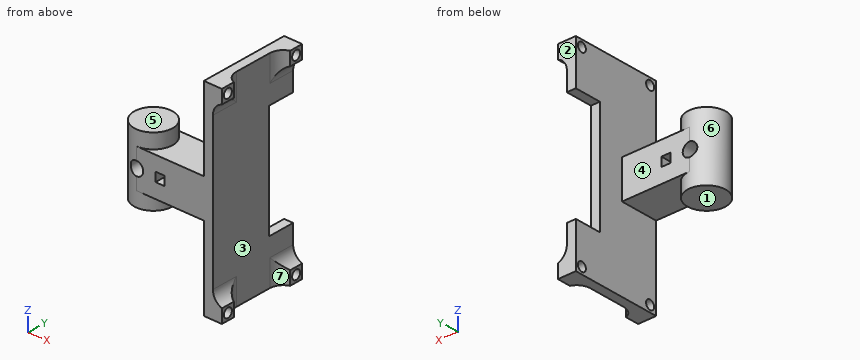
from build123d import *

# Parameters (mm, degrees)
SKETCH1_R               = 4.25
BOSS_EXTRUDE1_DEPTH     = 7.5
SKETCH2_W               = 8.5
SKETCH2_H               = 8.5
BOSS_EXTRUDE2_DEPTH     = 15
SKETCH3_W               = 45
SKETCH3_H               = 20
BOSS_EXTRUDE3_DEPTH     = 4
SKETCH4_R               = 1
CUT_EXTRUDE1_DEPTH      = 36.984371608
CUT_EXTRUDE2_DEPTH      = 2
SKETCH6_W               = 25
SKETCH6_H               = 6
CUT_EXTRUDE3_DEPTH      = 2
CUT_EXTRUDE4_DEPTH      = 32.614869919
CUT_EXTRUDE4_DEPTH_BACK = 32.614869919
SKETCH7_R               = 1.5
CUT_EXTRUDE5_DEPTH      = 34.396294705
CUT_EXTRUDE5_DEPTH_BACK = 34.396294705
SKETCH8_W               = 2
SKETCH8_H               = 2
FILLET1_R               = 3


with BuildPart() as part:
    # Sketch1 → Boss-Extrude1 (new, symmetric)
    with BuildSketch(Plane.XY):
        Circle(SKETCH1_R)
    extrude(amount=BOSS_EXTRUDE1_DEPTH, both=True)

    # Sketch2 → Boss-Extrude2 (add)
    with BuildSketch(Plane(origin=(0, 0, 0), x_dir=(0, 0, -1), z_dir=(1, 0, 0))):
        Rectangle(SKETCH2_W, SKETCH2_H)
    extrude(amount=BOSS_EXTRUDE2_DEPTH)

    # Sketch3 → Boss-Extrude3 (add)
    with BuildSketch(Plane(origin=(15, 0, 0), x_dir=(0, 0, -1), z_dir=(1, 0, 0))):
        with Locations((0, 5.75)):
            Rectangle(SKETCH3_W, SKETCH3_H)
    extrude(amount=BOSS_EXTRUDE3_DEPTH)

    # Sketch4 → Cut-Extrude1 (cut, through all)
    with BuildSketch(Plane(origin=(19, 0, 0), x_dir=(0, 0, -1), z_dir=(1, 0, 0))):
        with Locations((-21, 14.25)):
            Circle(SKETCH4_R)
        with Locations((-21, -2.75)):
            Circle(SKETCH4_R)
        with Locations((21, -2.75)):
            Circle(SKETCH4_R)
        with Locations((21, 14.25)):
            Circle(SKETCH4_R)
    extrude(amount=-CUT_EXTRUDE1_DEPTH, mode=Mode.SUBTRACT)

    # Sketch5 → Cut-Extrude2 (cut)
    with BuildSketch(Plane(origin=(19, 0, 0), x_dir=(0, 0, -1), z_dir=(1, 0, 0))):
        Polygon((19.5, 15.75), (-19.5, 15.75), (-19.5, 12.75), (-22.5, 12.75), (-22.5, -1.25), (-19.5, -1.25), (-19.5, -4.25), (19.5, -4.25), (19.5, -1.25), (22.5, -1.25), (22.5, 12.75), (19.5, 12.75), align=None)
    extrude(amount=-CUT_EXTRUDE2_DEPTH, mode=Mode.SUBTRACT)

    # Sketch6 → Cut-Extrude3 (cut)
    with BuildSketch(Plane(origin=(17, 0, 0), x_dir=(0, 0, -1), z_dir=(1, 0, 0))):
        with Locations((0, 12.75)):
            Rectangle(SKETCH6_W, SKETCH6_H)
    extrude(amount=-CUT_EXTRUDE3_DEPTH, mode=Mode.SUBTRACT)

    # Sketch7 → Cut-Extrude4 (cut, two sides: drawn at the far end of the back side and taken through both)
    with BuildSketch(Plane(origin=(0, 4.25, 0), x_dir=(1, 0, 0), z_dir=(0, 1, 0)).offset(-CUT_EXTRUDE4_DEPTH_BACK)):
        with Locations(Location((0, 0, 0), (0, 0, 270))):
            Circle(SKETCH7_R)
    extrude(amount=CUT_EXTRUDE4_DEPTH + CUT_EXTRUDE4_DEPTH_BACK, mode=Mode.SUBTRACT)

    # Sketch8 → Cut-Extrude5 (cut, two sides: drawn at the far end of the back side and taken through both)
    with BuildSketch(Plane(origin=(0, 0, 0), x_dir=(1, 0, 0), z_dir=(0, 1, 0)).offset(-CUT_EXTRUDE5_DEPTH_BACK)):
        with Locations((5.25, 0)):
            Rectangle(SKETCH8_W, SKETCH8_H)
    extrude(amount=CUT_EXTRUDE5_DEPTH + CUT_EXTRUDE5_DEPTH_BACK, mode=Mode.SUBTRACT)

    # Fillet1
    # the kernel refuses this fillet: 3 mm, written as the material it adds along each edge
    with BuildSketch(Plane(origin=(17, -1.25, -19.5), x_dir=(0, 1, 0), z_dir=(0, 0, -1)), Plane(origin=(17, -4.25, -19.5), x_dir=(0, 0, 1), z_dir=(0, 1, 0)), Plane(origin=(17, 12.75, -19.5), x_dir=(0, 0, 1), z_dir=(0, 1, 0)), Plane(origin=(17, 12.75, -22.5), x_dir=(0, -1, 0), z_dir=(0, 0, 1)), Plane(origin=(17, -1.25, 22.5), x_dir=(0, 1, 0), z_dir=(0, 0, -1)), Plane(origin=(17, 15.75, 19.5), x_dir=(0, 0, -1), z_dir=(0, -1, 0)), Plane(origin=(17, 12.75, 19.5), x_dir=(0, -1, 0), z_dir=(0, 0, 1))) as fillet1_piece_1:
        with BuildLine():
            CenterArc((2.828427125, 3), FILLET1_R, 199.471220634, 70.528779366)
            Line((0, 2), (-0.056568542, 1.98))
            ThreePointArc((-0.056568542, 1.98), (-0.06, 1), (-0.06, 0))
            Line((-0.06, 0), (0, -0.06))
            Line((0, -0.06), (2.828427125, -0.06))
            Line((2.828427125, -0.06), (2.828427125, 0))
        make_face()
    extrude(amount=3)
    with BuildSketch(Plane(origin=(17, -1.25, 19.5), x_dir=(1, 0, 0), z_dir=(0, -1, 0))) as fillet1_piece_2:
        with BuildLine():
            CenterArc((3, -2.828427125), FILLET1_R, 109.471220634, 70.528779366)
            Line((0, -2.828427125), (-0.06, -2.828427125))
            Line((-0.06, -2.828427125), (-0.06, 0))
            Line((-0.06, 0), (0, 0.06))
            ThreePointArc((0, 0.06), (1, 0.06), (1.98, 0.056568542))
            Line((1.98, 0.056568542), (2, 0))
        make_face()
    extrude(amount=3)
    with BuildSketch(Plane(origin=(17, -1.25, -12.428932188), x_dir=(0, 1, 0), z_dir=(0, 0, -1))) as fillet1_piece_3a_section:
        with BuildLine():
            CenterArc((2.828427125, 3), FILLET1_R, 199.471220634, 70.528779366)
            Line((0, 2), (-0.056568542, 1.98))
            ThreePointArc((-0.056568542, 1.98), (-0.06, 1), (-0.06, 0))
            Line((-0.06, 0), (0, -0.06))
            Line((0, -0.06), (2.828427125, -0.06))
            Line((2.828427125, -0.06), (2.828427125, 0))
        make_face()
    fillet1_piece_3a = extrude(amount=10.071067812, mode=Mode.PRIVATE)
    fillet1_piece_3a = split(fillet1_piece_3a, bisect_by=Plane(origin=(17.51353179, -0.571681569, -19.5), z_dir=(0, 0, 1)), keep=Keep.TOP, mode=Mode.PRIVATE)
    with BuildSketch(Plane(origin=(17, -4.25, -19.5), x_dir=(0, 0, 1), z_dir=(0, 1, 0))) as fillet1_piece_3b_section:
        with BuildLine():
            CenterArc((2.828427125, 3), FILLET1_R, 199.471220634, 70.528779366)
            Line((0, 2), (-0.056568542, 1.98))
            ThreePointArc((-0.056568542, 1.98), (-0.06, 1), (-0.06, 0))
            Line((-0.06, 0), (0, -0.06))
            Line((0, -0.06), (2.828427125, -0.06))
            Line((2.828427125, -0.06), (2.828427125, 0))
        make_face()
    fillet1_piece_3b = extrude(amount=10.071067812, mode=Mode.PRIVATE)
    fillet1_piece_3b = split(fillet1_piece_3b, bisect_by=Plane(origin=(17.51353179, -1.25, -18.821681569), z_dir=(0, 1, 0)), keep=Keep.TOP, mode=Mode.PRIVATE)
    fillet1_piece_3 = fillet1_piece_3a & fillet1_piece_3b
    add(fillet1_piece_3)
    with BuildSketch(Plane(origin=(17, 5.678932188, -19.5), x_dir=(0, 0, 1), z_dir=(0, 1, 0))) as fillet1_piece_4a_section:
        with BuildLine():
            CenterArc((2.828427125, 3), FILLET1_R, 199.471220634, 70.528779366)
            Line((0, 2), (-0.056568542, 1.98))
            ThreePointArc((-0.056568542, 1.98), (-0.06, 1), (-0.06, 0))
            Line((-0.06, 0), (0, -0.06))
            Line((0, -0.06), (2.828427125, -0.06))
            Line((2.828427125, -0.06), (2.828427125, 0))
        make_face()
    fillet1_piece_4a = extrude(amount=10.071067812, mode=Mode.PRIVATE)
    fillet1_piece_4a = split(fillet1_piece_4a, bisect_by=Plane(origin=(17.51353179, 12.75, -18.821681569), z_dir=(0, -1, 0)), keep=Keep.TOP, mode=Mode.PRIVATE)
    with BuildSketch(Plane(origin=(17, 12.75, -22.5), x_dir=(0, -1, 0), z_dir=(0, 0, 1))) as fillet1_piece_4b_section:
        with BuildLine():
            CenterArc((2.828427125, 3), FILLET1_R, 199.471220634, 70.528779366)
            Line((0, 2), (-0.056568542, 1.98))
            ThreePointArc((-0.056568542, 1.98), (-0.06, 1), (-0.06, 0))
            Line((-0.06, 0), (0, -0.06))
            Line((0, -0.06), (2.828427125, -0.06))
            Line((2.828427125, -0.06), (2.828427125, 0))
        make_face()
    fillet1_piece_4b = extrude(amount=10.071067812, mode=Mode.PRIVATE)
    fillet1_piece_4b = split(fillet1_piece_4b, bisect_by=Plane(origin=(17.51353179, 12.071681569, -12.5), z_dir=(0, 0, -1)), keep=Keep.TOP, mode=Mode.PRIVATE)
    fillet1_piece_4b = split(fillet1_piece_4b, bisect_by=Plane(origin=(17.51353179, 12.071681569, -19.5), z_dir=(0, 0, 1)), keep=Keep.TOP, mode=Mode.PRIVATE)
    fillet1_piece_4 = fillet1_piece_4a & fillet1_piece_4b
    add(fillet1_piece_4)
    with BuildSketch(Plane(origin=(17, 5.821067812, 19.5), x_dir=(1, 0, 0), z_dir=(0, -1, 0))) as fillet1_piece_5a_section:
        with BuildLine():
            CenterArc((3, -2.828427125), FILLET1_R, 109.471220634, 70.528779366)
            Line((0, -2.828427125), (-0.06, -2.828427125))
            Line((-0.06, -2.828427125), (-0.06, 0))
            Line((-0.06, 0), (0, 0.06))
            ThreePointArc((0, 0.06), (1, 0.06), (1.98, 0.056568542))
            Line((1.98, 0.056568542), (2, 0))
        make_face()
    fillet1_piece_5a = extrude(amount=10.071067812, mode=Mode.PRIVATE)
    fillet1_piece_5a = split(fillet1_piece_5a, bisect_by=Plane(origin=(17.51353179, -1.25, 18.821681569), z_dir=(0, 1, 0)), keep=Keep.TOP, mode=Mode.PRIVATE)
    with BuildSketch(Plane(origin=(17, -1.25, 22.5), x_dir=(0, 1, 0), z_dir=(0, 0, -1))) as fillet1_piece_5b_section:
        with BuildLine():
            CenterArc((2.828427125, 3), FILLET1_R, 199.471220634, 70.528779366)
            Line((0, 2), (-0.056568542, 1.98))
            ThreePointArc((-0.056568542, 1.98), (-0.06, 1), (-0.06, 0))
            Line((-0.06, 0), (0, -0.06))
            Line((0, -0.06), (2.828427125, -0.06))
            Line((2.828427125, -0.06), (2.828427125, 0))
        make_face()
    fillet1_piece_5b = extrude(amount=10.071067812, mode=Mode.PRIVATE)
    fillet1_piece_5b = split(fillet1_piece_5b, bisect_by=Plane(origin=(17.51353179, -0.571681569, 19.5), z_dir=(0, 0, -1)), keep=Keep.TOP, mode=Mode.PRIVATE)
    fillet1_piece_5 = fillet1_piece_5a & fillet1_piece_5b
    add(fillet1_piece_5)
    with BuildSketch(Plane(origin=(17, 12.75, 12.428932188), x_dir=(0, -1, 0), z_dir=(0, 0, 1))) as fillet1_piece_6a_section:
        with BuildLine():
            CenterArc((2.828427125, 3), FILLET1_R, 199.471220634, 70.528779366)
            Line((0, 2), (-0.056568542, 1.98))
            ThreePointArc((-0.056568542, 1.98), (-0.06, 1), (-0.06, 0))
            Line((-0.06, 0), (0, -0.06))
            Line((0, -0.06), (2.828427125, -0.06))
            Line((2.828427125, -0.06), (2.828427125, 0))
        make_face()
    fillet1_piece_6a = extrude(amount=10.071067812, mode=Mode.PRIVATE)
    fillet1_piece_6a = split(fillet1_piece_6a, bisect_by=Plane(origin=(17.51353179, 12.071681569, 12.5), z_dir=(0, 0, 1)), keep=Keep.TOP, mode=Mode.PRIVATE)
    fillet1_piece_6a = split(fillet1_piece_6a, bisect_by=Plane(origin=(17.51353179, 12.071681569, 19.5), z_dir=(0, 0, -1)), keep=Keep.TOP, mode=Mode.PRIVATE)
    with BuildSketch(Plane(origin=(17, 15.75, 19.5), x_dir=(0, 0, -1), z_dir=(0, -1, 0))) as fillet1_piece_6b_section:
        with BuildLine():
            CenterArc((2.828427125, 3), FILLET1_R, 199.471220634, 70.528779366)
            Line((0, 2), (-0.056568542, 1.98))
            ThreePointArc((-0.056568542, 1.98), (-0.06, 1), (-0.06, 0))
            Line((-0.06, 0), (0, -0.06))
            Line((0, -0.06), (2.828427125, -0.06))
            Line((2.828427125, -0.06), (2.828427125, 0))
        make_face()
    fillet1_piece_6b = extrude(amount=10.071067812, mode=Mode.PRIVATE)
    fillet1_piece_6b = split(fillet1_piece_6b, bisect_by=Plane(origin=(17.51353179, 12.75, 18.821681569), z_dir=(0, -1, 0)), keep=Keep.TOP, mode=Mode.PRIVATE)
    fillet1_piece_6 = fillet1_piece_6a & fillet1_piece_6b
    add(fillet1_piece_6)


solid = part.part
The listing builds one solid part. Answer for the finished solid, in the listing's coordinates (mm). Face numbers are marked on the shaded views. A direction names the side the tool comes from. Give positions to 0.01 mm unless a question says otherwise; leave off trailing zeros. Write each loop counter-clockwise with the first axis right and the second up, starting at its lowest first coordinate (ties: lowest second). Pieces come first, ordered by that corner, then holes. Notation, with made-up numbers: (89, -36.5) -> (147, -36.5) arc R22 cw to (147, -9.5) -> close; hole circle Ø3 at (-19.75, 44.5). An arc over 180 degrees is marked (long way). Use a Markdown table: item, result.
(1) Section B-B, the plane y = 13.75 is taken. Determine the outline of the cut face in (x, z).
Return value:
| item | result |
|---|---|
| outline | (15, -22.5) -> (19, -22.5) -> (19, -21.87) -> (15, -21.87) -> close; (15, -20.13) -> (19, -20.13) -> (19, -19.5) arc R3 cw to (17, -16.67) -> (17, -12.5) -> (15, -12.5) -> close; (15, 12.5) -> (17, 12.5) -> (17, 16.67) arc R3 cw to (19, 19.5) -> (19, 20.13) -> (15, 20.13) -> close; (15, 21.87) -> (19, 21.87) -> (19, 22.5) -> (15, 22.5) -> close |
(2) Determine the mould class of the marked faces 1, 2 and 3 for opening direction Z: released by +Z, released by -Z, zero draft, split by the parting line, or undercut.
Return value:
| item | result |
|---|---|
| face 1 | released by -Z |
| face 2 | zero draft |
| face 3 | undercut |
(3) For the marked faces 4, 5, 6 and 7, determine the directions among +Z, -Z, +X, -X, +Y, -Y from which every point of the face is accessible in a straight line to the end or side of a thin tool.
Return value:
| item | result |
|---|---|
| face 4 | +Z, -Z, -X, +Y |
| face 5 | +Z, -X, +Y, -Y |
| face 6 | none |
| face 7 | +Z, -Z, +X |
(4) Section C-C, the plane x = 16.5 is taken. Determine the outline of the cut face in (y, z).
Return value:
| item | result |
|---|---|
| outline | (-4.25, -22.5) -> (15.75, -22.5) -> (15.75, -12.5) -> (9.75, -12.5) -> (9.75, 12.5) -> (15.75, 12.5) -> (15.75, 22.5) -> (-4.25, 22.5) -> close; hole circle Ø2 at (-2.75, -21); hole circle Ø2 at (-2.75, 21); hole circle Ø2 at (14.25, -21); hole circle Ø2 at (14.25, 21) |
(5) Flat-ended cylindrical pins translate along their axes: P1, Ø12, axis at y = 4.5, z = 9, coming from the +X side; P2, Ø1, axis at x = 13, y = 8.5, coming from the +Z side; P3, Ø12, axis at y = -0.5, z = -13.5, coming from the +X side; P4, Ø1, axis at x = 5, y = -2, coming from the -Z side. Find the tip coordinate at first contact, or state that the pin passes through.
Return value:
| item | result |
|---|---|
| P1 | x = 17 |
| P2 | through |
| P3 | x = 18.89 |
| P4 | z = -4.25 |
(6) Section A-A, the plane z = -21 is taken. Determine the outline of the cut face in (x, y), then the cut area to 3 significant figures.
Return value:
| item | result |
|---|---|
| outline | (15, -4.25) -> (19, -4.25) -> (19, -3.75) -> (15, -3.75) -> close; (15, -1.75) -> (19, -1.75) -> (19, -1.25) arc R3 cw to (17, 1.58) -> (17, 9.92) arc R3 cw to (19, 12.75) -> (19, 13.25) -> (15, 13.25) -> close; (15, 15.25) -> (19, 15.25) -> (19, 15.75) -> (15, 15.75) -> close |
| area | 39.1 mm2 |
(7) Find the intervals of material crossed by probe 1 along Y at (x, z) = (16.9, -21); probe 2 along X at (y, z) = (0.5, 0); probe 3 along Y at (x, z) = (17.5, -21), in increasing order. Write a range as from..to.
Return value:
| item | result |
|---|---|
| probe 1 | -4.25..-3.75, -1.75..13.25, 15.25..15.75 |
| probe 2 | -4.22..-1.5, 1.5..4.25, 6.25..17 |
| probe 3 | -4.25..-3.75, -1.75..-0.08, 11.58..13.25, 15.25..15.75 |
(8) Section D-D, the plane z = 5.5 is taken. Determine the outline of the cut face in (x, y), then the cut area to 3 significant figures.
Return value:
| item | result |
|---|---|
| outline | circle Ø8.5 at (0, 0); (15, -4.25) -> (17, -4.25) -> (17, 9.75) -> (15, 9.75) -> close |
| area | 84.7 mm2 |
